Design review of the part built by this model. Coordinates are the model's own, in mm. Face numbers are marked on the shaded views. A direction names the side the tool comes from. Round coordinates to 2 decimals unless told otherwise and drop trailing zeros. Loops run counter-clockwise (first coordinate to the right, second up) from the corner with the lowest first, then second, coordinate; pieces in that order, holes last. Notation, with made-up numbers: (79.25, -3) - (83.25, -3) arc R5 ccw to (83.25, 3) - close; hole circle Ø8 at (22.25, 28.25). An arc over 180 degrees is marked (long way). Answer as CSV lines item,"result". Start each with the question number.
(1) Consider section D-D (y = -57). Give the boundary of the cut face in (x, z), and give its area (3 significant figures).
(2) For the marked faces 1 and 2, list the 3-axis set-ups (+Z, -Z, +X, -X, +Y, -Y) from which the entire face can be reached by the end or side of a thin tool; tool diameter is ignored.
(3) Wall thickness on L1, parallel to Y at x = 34.5, z = 256; L2, parallel to X at y = -0.45, z = 185.5; L3, parallel to X at y = -0.8, z = 10: over which ranges is each line inside the solid? List them lowest first.
(4) Consider section A-A (x = 24). Give the boundary of the cut face in (y, z).
(5) For P1, Ø6.5, axis at x = 125, z = 10, coming from the -Y side; P2, Ø0.5, axis at y = -0.5, z = 148.5, coming from the -X side; P3, Ø5, axis at x = 67.5, z = 185.5, coming from the +Y side; P4, Ø6, axis at x = -7.5, z = 173, coming from the -Y side, all flat-tipped, find the tip position at first contact; note any pin that passes through.
(6) Consider section B-B (z = 81). Give the boundary of the cut face in (x, y).
(7) Consider section C-C (x = 115.5). Give the boundary of the cut face in (y, z).
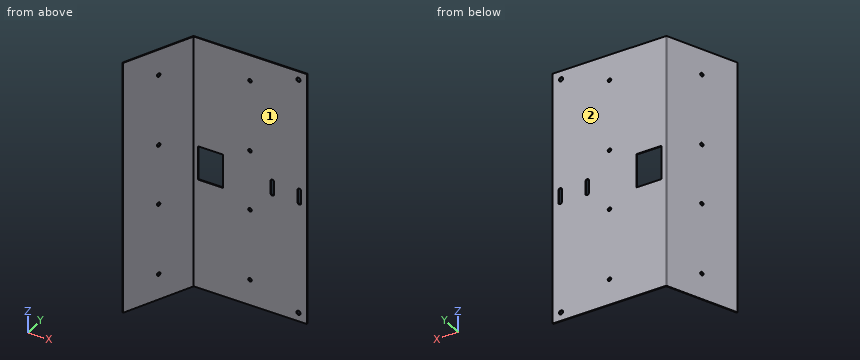
from build123d import *

# Parameters (mm, degrees)
T_LE_DE_BASE_PLI_E1_DEPTH = 300
ESQUISSE7_R               = 2.5
ENL_V_MAT_EXTRU_1_DEPTH   = 339.42205902
ENL_V_MAT_EXTRU_3_DEPTH   = 339.658074862
ESQUISSE14_W              = 30
ESQUISSE14_H              = 40
ENL_V_MAT_EXTRU_4_DEPTH   = 339.658074862
ESQUISSE15_R              = 2.1
ENL_V_MAT_EXTRU_5_DEPTH   = 339.658074862
ESQUISSE16_R              = 2.1
ENL_V_MAT_EXTRU_6_DEPTH   = 339.658074862


# Read off the part's stored shape, not the designer's step: Tôle de base pliée1
with BuildPart() as part:
    # Tôle de base pliée1 outline → Tôle de base pliée1 (new body)
    with BuildSketch(Plane.XY):
        with BuildLine():
            Line((-0.26214176, -0.599181166), (-35, -80))
            Line((-35, -80), (-34.083842665, -80.400818834))
            Line((-34.083842665, -80.400818834), (0.654015575, -1))
            Line((0.654015575, -1), (135, -1))
            Line((135, -1), (135, 0))
            Line((135, 0), (0.654015575, 0))
            ThreePointArc((0.654015575, 0), (0.10666689, -0.163095336), (-0.26214176, -0.599181166))
        make_face()
    extrude(amount=T_LE_DE_BASE_PLI_E1_DEPTH)

    # Esquisse7 → Enlèv. mat.-Extru.1 (cut, through all)
    with BuildSketch(Plane(origin=(0, -1, 0), x_dir=(-1, 0, 0), z_dir=(0, -1, 0))):
        with Locations(Location((-125, -290, 0), (0, 0, 90))):
            Circle(ESQUISSE7_R)
        with Locations(Location((-125, -10, 0), (0, 0, 90))):
            Circle(ESQUISSE7_R)
    extrude(amount=-ENL_V_MAT_EXTRU_1_DEPTH, mode=Mode.SUBTRACT)

    # Esquisse10 → Enlèv. mat.-Extru.3 (cut, through all)
    with BuildSketch(Plane(origin=(0, 0, 0), x_dir=(1, 0, 0), z_dir=(0, 1, 0))):
        with BuildLine():
            Line((96.1, -142.5), (96.1, -157.5))
            ThreePointArc((96.1, -157.5), (94, -159.6), (91.9, -157.5))
            Line((91.9, -157.5), (91.9, -142.5))
            ThreePointArc((91.9, -142.5), (94, -140.4), (96.1, -142.5))
        make_face()
        with BuildLine():
            Line((128.1, -142.5), (128.1, -157.5))
            ThreePointArc((128.1, -157.5), (126, -159.6), (123.9, -157.5))
            Line((123.9, -157.5), (123.9, -142.5))
            ThreePointArc((123.9, -142.5), (126, -140.4), (128.1, -142.5))
        make_face()
    extrude(amount=-ENL_V_MAT_EXTRU_3_DEPTH, mode=Mode.SUBTRACT)

    # Esquisse14 → Enlèv. mat.-Extru.4 (cut, through all)
    with BuildSketch(Plane(origin=(0, 0, 0), x_dir=(1, 0, 0), z_dir=(0, 1, 0))):
        with Locations((20.654015575, -150)):
            Rectangle(ESQUISSE14_W, ESQUISSE14_H)
    extrude(amount=-ENL_V_MAT_EXTRU_4_DEPTH, mode=Mode.SUBTRACT)

    # Esquisse15 → Enlèv. mat.-Extru.5 (cut, through all)
    with BuildSketch(Plane(origin=(0, 0, 0), x_dir=(1, 0, 0), z_dir=(0, 1, 0))):
        with Locations(Location((67.5, -114.5, 0), (0, 0, 270))):
            Circle(ESQUISSE15_R)
        with Locations(Location((67.5, -30.5, 0), (0, 0, 270))):
            Circle(ESQUISSE15_R)
        with Locations(Location((67.5, -269.5, 0), (0, 0, 270))):
            Circle(ESQUISSE15_R)
        with Locations(Location((67.5, -185.5, 0), (0, 0, 270))):
            Circle(ESQUISSE15_R)
    extrude(amount=-ENL_V_MAT_EXTRU_5_DEPTH, mode=Mode.SUBTRACT)

    # Esquisse16 → Enlèv. mat.-Extru.6 (cut, through all)
    with BuildSketch(Plane(origin=(0, 0, 0), x_dir=(0, 0, 1), z_dir=(-0.9161573349021892, 0.40081883401970764, 0))):
        with Locations(Location((114.5, -43.660622991, 0), (0, 0, 270))):
            Circle(ESQUISSE16_R)
        with Locations(Location((30.5, -43.660622991, 0), (0, 0, 270))):
            Circle(ESQUISSE16_R)
        with Locations(Location((269.5, -43.660622991, 0), (0, 0, 90))):
            Circle(ESQUISSE16_R)
        with Locations(Location((185.5, -43.660622991, 0), (0, 0, 90))):
            Circle(ESQUISSE16_R)
    extrude(amount=-ENL_V_MAT_EXTRU_6_DEPTH, mode=Mode.SUBTRACT)


solid = part.part
Determined:
1,outline,"(-24.94, 0) - (-23.85, 0) - (-23.85, 300) - (-24.94, 300) - close"
1,area,"327 mm^2"
2,face 1,"+Z, -Z, +X, -Y"
2,face 2,"+Z, -Z, +X, -X, +Y"
3,L1,"y = -1 to 0"
3,L2,"x = -0.18 to 65.4, 69.6 to 135"
3,L3,"x = -0.35 to 122.5, 127.5 to 135"
4,outline,"(-1, 0) - (0, 0) - (0, 130) - (-1, 130) - close; (-1, 170) - (0, 170) - (0, 300) - (-1, 300) - close"
5,P1,"stops at y = -1"
5,P2,"stops at x = -0.33"
5,P3,"stops at y = 0"
5,P4,"stops at y = -26.49"
6,outline,"(-35, -80) - (-34.08, -80.4) - (0.65, -1) - (135, -1) - (135, 0) - (0.65, 0) arc R1 ccw to (-0.26, -0.6) - close"
7,outline,"(-1, 0) - (0, 0) - (0, 300) - (-1, 300) - close"
